Geometry: final body of the model. Coordinates: model frame, mm. A direction names the side the tool comes from. Round coordinates to 2 decimals unless told otherwise and drop trailing zeros. Order: outer loops, then holes, each group sorted by start corner. A loop starts at its lowest first (then second) coordinate and runs counter-clockwise, first axis right, second up. Notation, with made-up numbers: (85, 53.5) -> (131, 53.5) arc R21 ccw to (131, 77.5) -> close; hole circle Ø10 at (75, -19). An arc over 180 degrees is marked (long way). Put each result on its own line as item: value.
Autodesk Inventor part; units mm, degrees
ref_plane "YZ Plane" through (0, 0, 0) normal (1, 0, 0) x (0, 1, 0)
ref_plane "XZ Plane" through (0, 0, 0) normal (0, 1, 0) x (-1, 0, 0)
ref_plane "XY Plane" through (0, 0, 0) normal (0, 0, 1) x (1, 0, 0)
sketch "Skizze1" plane through (0, 0, 0) normal (0, 0, 1) x (1, 0, 0)
  circle A0 centre (0, 0) radius 12.3
  arc A1 (13.4907, -0.4999) -> (13.4907, 0.4999) centre (13.5, 0) ccw
  arc A2 (-13.4907, -0.4999) -> (13.4907, -0.4999) centre (0, 0) ccw
  line L0 (0, -18.9) -> (0, 18.9) construction
  line L1 (-20.7866, 0) -> (20.7866, 0) construction
  arc A3 (7.1783, 11.4334) -> (6.3124, 11.9333) centre (6.75, 11.6913) ccw
  arc A4 (-6.3124, 11.9333) -> (-7.1783, 11.4334) centre (-6.75, 11.6913) ccw
  arc A5 (-13.4907, 0.4999) -> (-13.4907, -0.4999) centre (-13.5, 0) ccw
  arc A6 (-7.1783, -11.4334) -> (-6.3124, -11.9333) centre (-6.75, -11.6913) ccw
  arc A7 (6.3124, -11.9333) -> (7.1783, -11.4334) centre (6.75, -11.6913) ccw
  arc A8 (13.4907, 0.4999) -> (7.1783, 11.4334) centre (0, 0) ccw
  arc A9 (6.3124, 11.9333) -> (-6.3124, 11.9333) centre (0, 0) ccw
  arc A10 (-7.1783, 11.4334) -> (-13.4907, 0.4999) centre (0, 0) ccw
  point P0 (-13.4907, -0.4999)
  point P1 (-6.3124, -11.9333)
  dimension "d3" = 0
  dimension "d7" = 1
  dimension "d9" = 13.5
  dimension "d10" = 24.6
  dimension "d11" = 13.5
  dimension "d12" = 0
  dimension "d13" = 13.4907
  dimension "d14" = 13.4907
  dimension "d69" = 360
extrude "Extrusion1" add sketch "Skizze1" along normal blind 1.8
sketch "Skizze2" plane through (0, 0, 1.8) normal (0, 0, 1) x (1, 0, 0)
  circle A0 centre (0, 0) radius 16
  dimension "d15" = 32
extrude "Extrusion2" add sketch "Skizze2" along normal blind 1.2
properties part number "Lid_plain" material "PC/ABS-Kunststoff"
1. Cut plane B-B on x = -4. Return loops of the section in (y, z).
Ans:
outline: (-15.49, 1.8) -> (-12.89, 1.8) -> (-12.89, 0) -> (-11.63, 0) -> (-11.63, 1.8) -> (11.63, 1.8) -> (11.63, 0) -> (12.89, 0) -> (12.89, 1.8) -> (15.49, 1.8) -> (15.49, 3) -> (-15.49, 3) -> close
2. Draft query along X for faces 6 (the face through (11.737, -6.67, 0.887)), 7 (the face through (-11.737, 6.67, 0.887)), 8 (the face through (-7.01, 12.12, 0.89)), 9 (the face through (6.99, 12.13, 0.89)). Return one class per face: +X half, -X half, draft (parallel to the pull), parting line (faces both ways), or undercut.
Ans:
face 6: +X half
face 7: -X half
face 8: undercut
face 9: undercut
3. Material intervals for probe 1 along Y at (x, z) = (0, 1.1); probe 2 along Z at (x, y) = (-15, 4); probe 3 along X at (y, z) = (6, 0.8), sorted ascending.
Ans:
probe 1: -13.5 to -12.3, 12.3 to 13.5
probe 2: 1.8 to 3
probe 3: -12.09 to -10.74, 10.74 to 12.09
4. Cut plane A-A on y = 0. Return loops of the section in (x, z).
Ans:
outline: (-16, 1.8) -> (-14, 1.8) -> (-14, 0) -> (-12.3, 0) -> (-12.3, 1.8) -> (12.3, 1.8) -> (12.3, 0) -> (14, 0) -> (14, 1.8) -> (16, 1.8) -> (16, 3) -> (-16, 3) -> close
5. Set-up query: faces 1 (the face through (-0.1, 13.5, 0.9)), 2 (the face through (0, 0, 3)), 3 (the face through (-11.5, -4.9, 0)), 4 (the face through (0.1, -13.5, 0.9)), 5 (the face through (0, 0, 1.8)). Return all of +Z, -Z, +X, -X, +Y, -Y with unobstructed straight access to the full face (end or side cutting, diameter ignored); none if empty.
Ans:
face 1: -Z, +Y
face 2: +Z, +X, -X, +Y, -Y
face 3: -Z, +X, -X, +Y, -Y
face 4: -Z, -Y
face 5: -Z
6. Contact query for flat-ended pins moving along their axis: P1, Ø3, axis at x = 3, y = -3.5, coming from the -Z side; P2, Ø1.5, axis at x = -12, z = 2, coming from the +Y side. Output: stop coordinate, or through.
Ans:
P1: z = 1.8
P2: y = 11.38
